Design review of the part built by this model. Coordinates are the model's own, in mm. Face numbers are marked on the shaded views. Give positions to 0.01 mm unless a question says otherwise; leave off trailing zeros. Write each loop counter-clockwise with the first axis right and the second up, starting at its lowest first coordinate (ties: lowest second). Pieces come first, ordered by that corner, then holes. Notation, with made-up numbers: (11.25, 57.5) - (47.25, 57.5) arc R35 ccw to (47.25, 89.5) - close; hole circle Ø7 at (-30, 40). An arc over 180 degrees is marked (long way). Use a Markdown table: item, result. Add a question column.
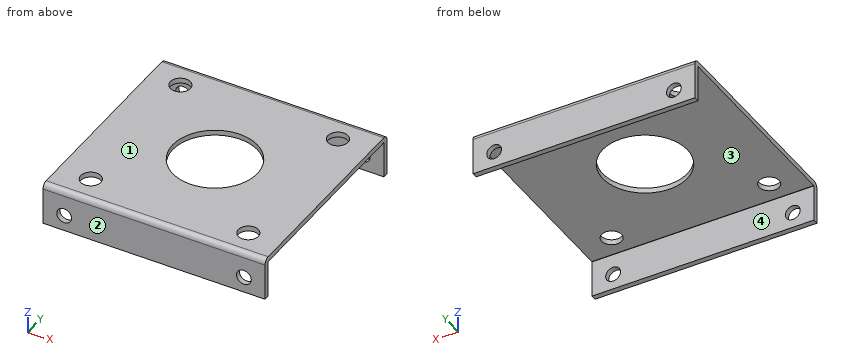
```python
from build123d import *

# Parameters (mm, degrees)
SKETCH1_W                    = 210
SKETCH1_H                    = 200
BASE_FLANGE1_DEPTH           = 5
EDGE_FLANGE1_STRIP_W         = 20.4
EDGE_FLANGE1_STRIP_H         = 5
EDGE_FLANGE1_STRIP_CUT_DEPTH = 210
EDGE_FLANGE1_DEPTH           = 210
EDGE_FLANGE2_STRIP_W         = 20.4
EDGE_FLANGE2_STRIP_H         = 5
EDGE_FLANGE2_STRIP_CUT_DEPTH = 210
EDGE_FLANGE2_DEPTH           = 210
CUT_EXTRUDE1_DEPTH           = 151.416089565
CUT_EXTRUDE1_DEPTH_BACK      = 151.416089565
SKETCH12_R                   = 40
CUT_EXTRUDE2_DEPTH           = 151.416089565
CUT_EXTRUDE2_DEPTH_BACK      = 151.416089565
SKETCH13_R                   = 9.5
CUT_EXTRUDE3_DEPTH           = 230.401394939
CUT_EXTRUDE3_DEPTH_BACK      = 230.401394939
SKETCH14_R                   = 7


# Sheet-metal steps are written as plain solids
with BuildPart() as part:
    # Sketch1 → Base-Flange1 (new body)
    with BuildSketch(Plane.XY):
        Rectangle(SKETCH1_W, SKETCH1_H)
    extrude(amount=-BASE_FLANGE1_DEPTH)

    # Edge-Flange1 strip (across the edge) → Edge-Flange1 strip cut (cut)
    with BuildSketch(Plane(origin=(-105, 100, -5), x_dir=(0, -1, 0), z_dir=(1, 0, 0))):
        with Locations((-5, -2.5)):
            Rectangle(EDGE_FLANGE1_STRIP_W, EDGE_FLANGE1_STRIP_H)
    extrude(amount=EDGE_FLANGE1_STRIP_CUT_DEPTH, mode=Mode.SUBTRACT)

    # Edge-Flange1 section (across the edge) → Edge-Flange1 (add)
    with BuildSketch(Plane(origin=(-105, 100, -5), x_dir=(0, -1, 0), z_dir=(1, 0, 0))):
        with BuildLine():
            Line((0, 0.2), (0, 35))
            Line((0, 35), (5, 35))
            Line((5, 35), (5, 0.2))
            ThreePointArc((5, 0.2), (5.058578644, 0.058578644), (5.2, 0))
            Line((5.2, 0), (5.2, -5))
            ThreePointArc((5.2, -5), (1.523044738, -3.476955262), (0, 0.2))
        make_face()
    extrude(amount=EDGE_FLANGE1_DEPTH)

    # Edge-Flange2 strip (across the edge) → Edge-Flange2 strip cut (cut)
    with BuildSketch(Plane(origin=(105, -100, -5), x_dir=(0, 1, 0), z_dir=(-1, 0, 0))):
        with Locations((-5, -2.5)):
            Rectangle(EDGE_FLANGE2_STRIP_W, EDGE_FLANGE2_STRIP_H)
    extrude(amount=EDGE_FLANGE2_STRIP_CUT_DEPTH, mode=Mode.SUBTRACT)

    # Edge-Flange2 section (across the edge) → Edge-Flange2 (add)
    with BuildSketch(Plane(origin=(105, -100, -5), x_dir=(0, 1, 0), z_dir=(-1, 0, 0))):
        with BuildLine():
            Line((0, 0.2), (0, 35))
            Line((0, 35), (5, 35))
            Line((5, 35), (5, 0.2))
            ThreePointArc((5, 0.2), (5.058578644, 0.058578644), (5.2, 0))
            Line((5.2, 0), (5.2, -5))
            ThreePointArc((5.2, -5), (1.523044738, -3.476955262), (0, 0.2))
        make_face()
    extrude(amount=EDGE_FLANGE2_DEPTH)

    # Sketch12 → Cut-Extrude1 (cut, two sides: drawn at the far end of the back side and taken through both)
    with BuildSketch(Plane.XY.offset(-CUT_EXTRUDE1_DEPTH_BACK)):
        with Locations(Location((0, 0, 0), (0, 0, 180))):
            Circle(SKETCH12_R)
    extrude(amount=CUT_EXTRUDE1_DEPTH + CUT_EXTRUDE1_DEPTH_BACK, mode=Mode.SUBTRACT)

    # Sketch13 → Cut-Extrude2 (cut, two sides: drawn at the far end of the back side and taken through both)
    with BuildSketch(Plane.XY.offset(-CUT_EXTRUDE2_DEPTH_BACK)):
        with Locations(Location((73.282986518, 74.49502971, 0), (0, 0, 180))):
            Circle(SKETCH13_R)
        with Locations(Location((-75.717013482, 74.49502971, 0), (0, 0, 180))):
            Circle(SKETCH13_R)
        with Locations(Location((-74.5, -74.5, 0), (0, 0, 180))):
            Circle(SKETCH13_R)
        with Locations(Location((74.5, -74.5, 0), (0, 0, 180))):
            Circle(SKETCH13_R)
    extrude(amount=CUT_EXTRUDE2_DEPTH + CUT_EXTRUDE2_DEPTH_BACK, mode=Mode.SUBTRACT)

    # Sketch14 → Cut-Extrude3 (cut, two sides: drawn at the far end of the back side and taken through both)
    with BuildSketch(Plane(origin=(0, -100, 0), x_dir=(-1, 0, 0), z_dir=(0, -1, 0)).offset(-CUT_EXTRUDE3_DEPTH_BACK)):
        with Locations(Location((85, 25, 0), (0, 0, 270))):
            Circle(SKETCH14_R)
        with Locations(Location((-85, 25, 0), (0, 0, 270))):
            Circle(SKETCH14_R)
    extrude(amount=CUT_EXTRUDE3_DEPTH + CUT_EXTRUDE3_DEPTH_BACK, mode=Mode.SUBTRACT)


solid = part.part
```
(1) Mouldability with a two-part tool opening along Y and no side actions: class the marked faces 1, 2, 3 and 4 as +Y half, -Y half, draft (parallel to the pull), parting line (faces both ways), or undercut.
(2) Insertion check: pin 1 (22 mm diameter, centred on x = -75.72, y = 74.5, fed in from -Z). The pin has a flat end and moves straight along its axis. Give the tip position at first contact, or say it passes through.
(3) Add section D-D (z = -37). State the section outline as (x, y) points.
(4) For line 1 along X through (y, z) = (-98.9, -25); line 2 along X through (y, z) = (-74, -1); line 3 along Y through (x, z) = (44, -32), list the stretches that pass through material, from the lowest coordinate up.
(5) Add section C-C (y = -68.5). State the section outline as (x, z) points, and give its area (3 significant figures).
(6) Add section A-A (z = -25). State the section outline as (x, y) points, and give its area (3 significant figures).
(7) Add section B-B (x = 0). State the section outline as (y, z) points, and give its area (3 significant figures).
Answers follow:
| question | item | result |
|---|---|---|
| 1 | face 1 | draft |
| 1 | face 2 | -Y half |
| 1 | face 3 | undercut |
| 1 | face 4 | undercut |
| 2 | pin 1 | z = -5 |
| 3 | outline | (-105, -100) - (105, -100) - (105, -95) - (-105, -95) - close; (-105, 95) - (105, 95) - (105, 100) - (-105, 100) - close |
| 4 | line 1 | -105 to -92, -78 to 78, 92 to 105 |
| 4 | line 2 | -105 to -83.99, -65.01 to 65.01, 83.99 to 105 |
| 4 | line 3 | -100 to -95, 95 to 100 |
| 5 | outline | (-105, -5) - (-81.87, -5) - (-81.87, 0) - (-105, 0) - close; (-67.13, -5) - (67.13, -5) - (67.13, 0) - (-67.13, 0) - close; (81.87, -5) - (105, -5) - (105, 0) - (81.87, 0) - close |
| 5 | area | 903 mm^2 |
| 6 | outline | (-105, -100) - (-92, -100) - (-92, -95) - (-105, -95) - close; (-105, 95) - (-92, 95) - (-92, 100) - (-105, 100) - close; (-78, -100) - (78, -100) - (78, -95) - (-78, -95) - close; (-78, 95) - (78, 95) - (78, 100) - (-78, 100) - close; (92, -100) - (105, -100) - (105, -95) - (92, -95) - close; (92, 95) - (105, 95) - (105, 100) - (92, 100) - close |
| 6 | area | 1,820 mm^2 |
| 7 | outline | (-100, -40) - (-95, -40) - (-95, -5.2) arc R0.2 cw to (-94.8, -5) - (-40, -5) - (-40, 0) - (-94.8, 0) arc R5.2 ccw to (-100, -5.2) - close; (40, -5) - (94.8, -5) arc R0.2 cw to (95, -5.2) - (95, -40) - (100, -40) - (100, -5.2) arc R5.2 ccw to (94.8, 0) - (40, 0) - close |
| 7 | area | 938 mm^2 |
